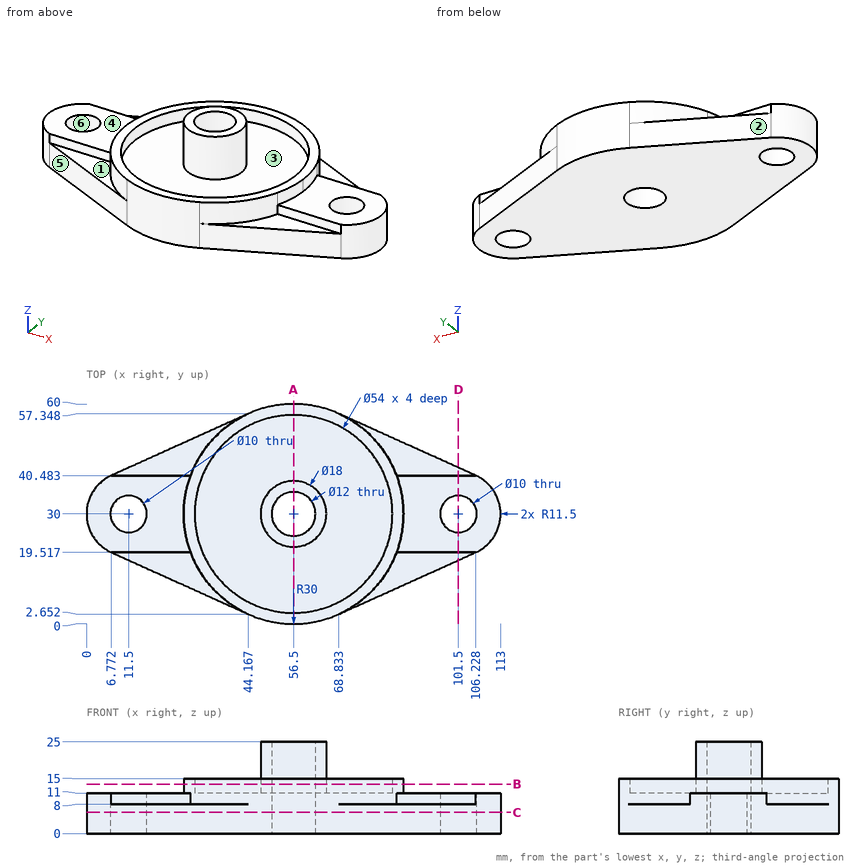
Geometry check sheet. Reference: drawing and pictorial views, mm from the part's lowest x, y, z. A direction names the side the tool comes from. Coordinates: 2 decimals unless noted, no trailing zeros. Write each loop counter-clockwise with the first axis right and the second up, starting at its lowest first coordinate (ties: lowest second). Pieces come first, ordered by that corner, then holes. Notation, with made-up numbers: (-39, 26.25) - (-29, 26.25) arc R18 cw to (-29, 48.25) - close; hole circle Ø2 at (9, 65). An arc over 180 degrees is marked (long way). One line per question, with ' | ' between items. Start each with the question number.
1. Material ranges on line 1 along Y through (x, z) = (56, 14) (1 decimal); line 2 along X through (y, z) = (25, 14.25) (1 decimal); line 3 along Z through (x, y) = (79, 13.5), recorded low to high.
2. Draft check along Y on the marked faces 4, 5 and 6. Enter one of: released by +Y, released by -Y, zero draft, split by the parting line, or undercut.
3. Access from +Z, -Z, +X, -X, +Y, -Y to the whole of each face (thin tool, end or side, straight path). Record for the marked faces 1, 2 and 3.
4. Section check C-C (z = 5.75). Enter the section's corners in (x, y), plus the area to 3 significant figures.
5. Section check D-D (x = 101.5). Enter the section's corners in (y, z) (1 decimal).
6. Gauge pin test, flat ends, axial feed: P1, Ø3, axis at y = 28, z = 21.5, coming from the -X side; P2, Ø23, axis at x = 15.5, y = 27.5, coming from the +Z side; P3, Ø0.9, axis at x = 100, z = 9.5, coming from the -Y side. Record the tip position at first contact, or that the pin passes through.
7. Section check B-B (z = 13.5). Enter the section's corners in (x, y).
8. Section check A-A (x = 56.5). Enter the section's corners in (y, z), plus the area to 3 significant figures.
Computed values:
1) line 1: 0 to 3, 21 to 24, 36 to 39, 57 to 60 | line 2: 26.9 to 30, 49 to 53.2, 59.8 to 64, 83 to 86.1 | line 3: 0 to 15
2) face 4: zero draft | face 5: released by -Y | face 6: undercut
3) face 1: +Z, -X, -Y | face 2: +Z, -Z, -X, +Y | face 3: +Z
4) outline: (6.77, 19.52) - (44.17, 2.65) arc R30 ccw to (68.83, 2.65) - (106.23, 19.52) arc R11.5 ccw to (106.23, 40.48) - (68.83, 57.35) arc R30 ccw to (44.17, 57.35) - (6.77, 40.48) arc R11.5 ccw to start; hole circle Ø10 at (11.5, 30); hole circle Ø12 at (56.5, 30); hole circle Ø10 at (101.5, 30) | area: 4,200 mm²
5) outline: (17.4, 0) - (25, 0) - (25, 11) - (19.5, 11) - (19.5, 8) - (17.4, 8) - close; (35, 0) - (42.6, 0) - (42.6, 8) - (40.5, 8) - (40.5, 11) - (35, 11) - close
6) P1: x = 47.51 | P2: z = 15 | P3: y = 19.52
7) outline: (28.39, 19.52) arc R30 ccw to (44.17, 2.65) arc R30 ccw to (68.83, 2.65) arc R30 ccw to (84.61, 19.52) arc R30 ccw to (86.5, 30) arc R30 ccw to (84.61, 40.48) arc R30 ccw to (68.83, 57.35) arc R30 ccw to (44.17, 57.35) arc R30 ccw to (28.39, 40.48) arc R30 ccw to start; circle Ø18 at (56.5, 30); hole circle Ø54 at (56.5, 30); hole circle Ø12 at (56.5, 30)
8) outline: (0, 0) - (24, 0) - (24, 25) - (21, 25) - (21, 11) - (3, 11) - (3, 15) - (0, 15) - close; (36, 0) - (60, 0) - (60, 15) - (57, 15) - (57, 11) - (39, 11) - (39, 25) - (36, 25) - close | area: 636 mm²
